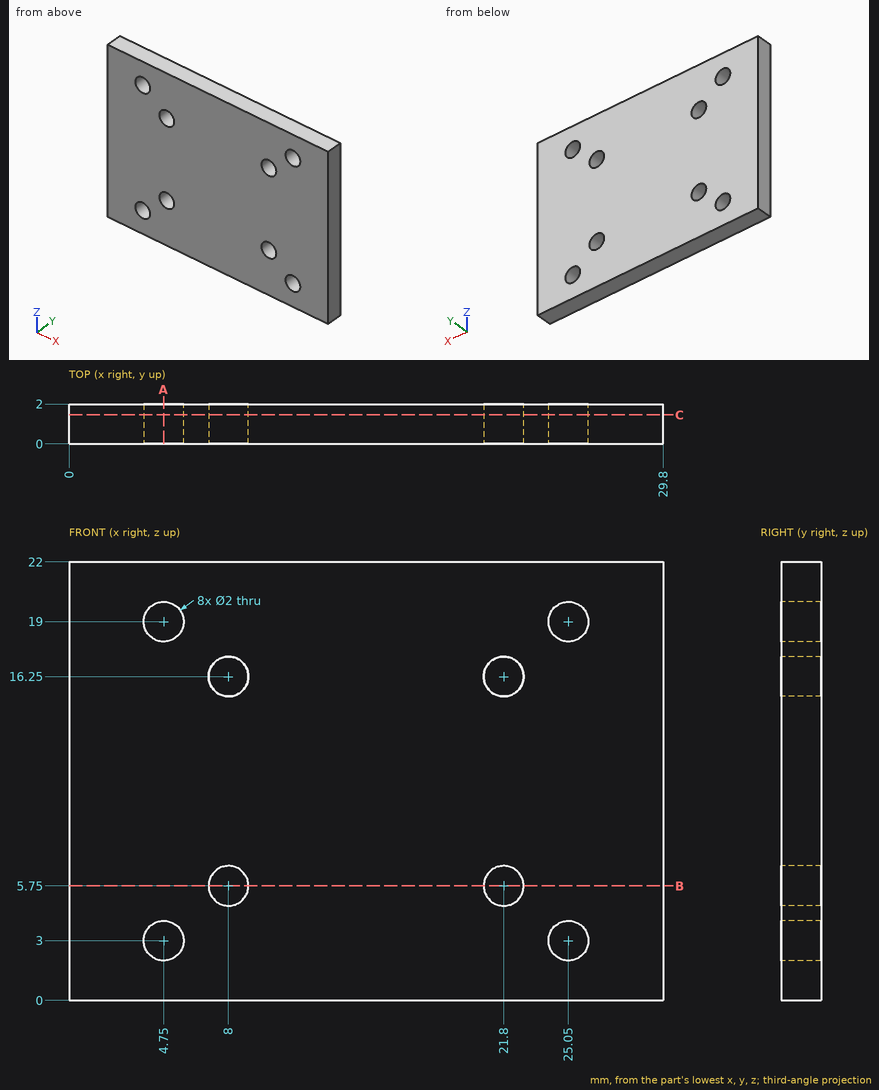
Here's the drawing with two shaded views (mm, measured from the low corner). I have some questions. Round coordinates to 2 decimals unless told otherwise and drop trailing zeros. Loops run counter-clockwise (first coordinate to the right, second up) from the corner with the lowest first, then second, coordinate; pieces in that order, holes last.
Item 1: Suppose I cut it at B-B, the plane z = 5.75. Write out the boundary of the cut face in (x, y), then the cut area to 3 significant figures.
Item 2: Suppose I cut it at C-C, the plane y = 1.45. State how many separate pieces and enclosed holes the cut face has, then the cut area to 3 significant figures.
Item 3: Please list where these lines run through material, in increasing order: L1, parallel to Z at x = 4.75, y = 0.85; L2, parallel to X at y = 0.85, z = 3; L3, parallel to X at y = 1.25, z = 16.25.
Item 4: Suppose I cut it at A-A, the plane x = 4.75. Write out the boundary of the cut face in (y, z), then the cut area to 3 significant figures.
Reported:
1. outline: (0, 0) - (7, 0) - (7, 2) - (0, 2) - close; (9, 0) - (20.8, 0) - (20.8, 2) - (9, 2) - close; (22.8, 0) - (29.8, 0) - (29.8, 2) - (22.8, 2) - close
1. area: 51.6 mm2
2. separate pieces: 1
2. enclosed holes: 8
2. area: 630 mm2
3. L1: z = 0 to 2, 4 to 18, 20 to 22
3. L2: x = 0 to 3.75, 5.75 to 24.05, 26.05 to 29.8
3. L3: x = 0 to 7, 9 to 20.8, 22.8 to 29.8
4. outline: (0, 0) - (2, 0) - (2, 2) - (0, 2) - close; (0, 4) - (2, 4) - (2, 18) - (0, 18) - close; (0, 20) - (2, 20) - (2, 22) - (0, 22) - close
4. area: 36.0 mm2
